Here's how the part is built. I have some questions about the finished solid (model axes, mm). Face numbers are marked on the shaded views. Give positions to 0.01 mm unless a question says otherwise; leave off trailing zeros. Order: outer loops, then holes, each group sorted by start corner. A loop starts at its lowest first (then second) coordinate and runs counter-clockwise, first axis right, second up. Notation, with made-up numbers: (42, 63) -> (85, 63) arc R12 cw to (85, 78) -> close; hole circle Ø8 at (70, 19.25). An arc over 180 degrees is marked (long way). Write each question's results on one line, items separated by ' | '. Start each with the question number.
Q1. Imagine slicing it at A-A, the plane z = 28. Please give me the cut outline in (x, y), then the cut area to 3 significant figures.
Q2. I'm going to push flat-ended pins straight in: pin 1 (1.4 mm diameter, centred on x = 6, y = -11.5, fed in from -Z); pin 2 (3 mm diameter, centred on y = -7, z = -16.5, fed in from -X); pin 3 (6.5 mm diameter, centred on x = 2, z = -47.5, fed in from -Y); pin 4 (1.5 mm diameter, centred on x = -12.5, z = 13, fed in from +Y). Where does each tip first touch, or does it pass through?
Q3. Imagine slicing it at B-B, the plane z = -23.5. Please give me the cut outline in (x, y).
Q4. Thinking about a two-plate mould opening in X: for the marked faces 1 and 2, which applies, pulls with the +X half, pulls with the -X half, needs draft (parallel to the pull), parting line crosses it, or undercut?
Q5. I need wall thicknesses on line 1 along Y through (x, z) = (-19.5, 1); line 2 along X through (y, z) = (-11.75, -6); line 3 along X through (y, z) = (-10, -40.5). Which ranges of each line are inside material? Lowest first, please. Write a range as [from, to].
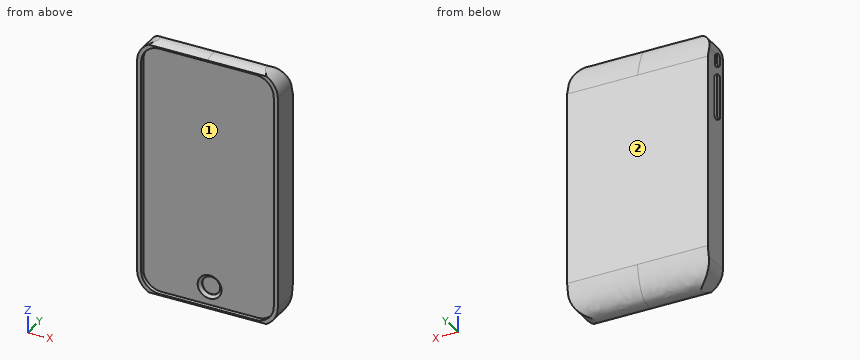
```python
from build123d import *

# Parameters (mm, degrees)
F0_R     = 3.9502971089
F1_DEPTH = 10.668
F2_DEPTH = 12.446
F3_START = 9.144
F3_DEPTH = 9.906
F4_SIZE  = 1.27
F6_DEPTH = 34.798
F8_DEPTH = 31.75


with BuildPart() as f1:
    # F0 (on Front) → F1 (new body)
    with BuildSketch(Plane.XZ):
        with BuildLine():
            Line((-20.9762947197, -56.8147292361), (20.9762947197, -56.8147292361))
            ThreePointArc((20.9762947197, -56.8147292361), (27.8910919329, -53.9505264493), (30.7552947197, -47.0357292361))
            Line((30.7552947197, -47.0357292361), (30.7552947197, 47.0357292361))
            ThreePointArc((30.7552947197, 47.0357292361), (27.8910919329, 53.9505264493), (20.9762947197, 56.8147292361))
            Line((20.9762947197, 56.8147292361), (-20.9762947197, 56.8147292361))
            ThreePointArc((-20.9762947197, 56.8147292361), (-27.8910919329, 53.9505264493), (-30.7552947197, 47.0357292361))
            Line((-30.7552947197, 47.0357292361), (-30.7552947197, -47.0357292361))
            ThreePointArc((-30.7552947197, -47.0357292361), (-27.8910919329, -53.9505264493), (-20.9762947197, -56.8147292361))
        make_face()
        with BuildLine():
            ThreePointArc((20.9762947197, 55.0367310643), (26.6338573688, 52.6932918851), (28.977296548, 47.0357292361))
            Line((28.977296548, 47.0357292361), (28.977296548, -47.0357292361))
            ThreePointArc((28.977296548, -47.0357292361), (26.6338573688, -52.6932918851), (20.9762947197, -55.0367310643))
            Line((20.9762947197, -55.0367310643), (-20.9762947197, -55.0367310643))
            ThreePointArc((-20.9762947197, -55.0367310643), (-26.6338573688, -52.6932918851), (-28.977296548, -47.0357292361))
            Line((-28.977296548, -47.0357292361), (-28.977296548, 47.0357292361))
            ThreePointArc((-28.977296548, 47.0357292361), (-26.6338573688, 52.6932918851), (-20.9762947197, 55.0367310643))
            Line((-20.9762947197, 55.0367310643), (20.9762947197, 55.0367310643))
        make_face(mode=Mode.SUBTRACT)
        with BuildLine():
            Line((28.977296548, -47.0357292361), (28.977296548, 47.0357292361))
            ThreePointArc((28.977296548, 47.0357292361), (26.6338573688, 52.6932918851), (20.9762947197, 55.0367310643))
            Line((20.9762947197, 55.0367310643), (-20.9762947197, 55.0367310643))
            ThreePointArc((-20.9762947197, 55.0367310643), (-26.6338573688, 52.6932918851), (-28.977296548, 47.0357292361))
            Line((-28.977296548, 47.0357292361), (-28.977296548, -47.0357292361))
            ThreePointArc((-28.977296548, -47.0357292361), (-26.6338573688, -52.6932918851), (-20.9762947197, -55.0367310643))
            Line((-20.9762947197, -55.0367310643), (20.9762947197, -55.0367310643))
            ThreePointArc((20.9762947197, -55.0367310643), (26.6338573688, -52.6932918851), (28.977296548, -47.0357292361))
        make_face()
        with Locations((0, -47.0412708819)):
            Circle(F0_R, mode=Mode.SUBTRACT)
        with Locations((0, -47.0412708819)):
            Circle(F0_R)
    extrude(amount=F1_DEPTH)

    # F0 (on Front) → F2 (join)
    with BuildSketch(Plane.XZ):
        with BuildLine():
            Line((-20.9762947197, -56.8147292361), (20.9762947197, -56.8147292361))
            ThreePointArc((20.9762947197, -56.8147292361), (27.8910919329, -53.9505264493), (30.7552947197, -47.0357292361))
            Line((30.7552947197, -47.0357292361), (30.7552947197, 47.0357292361))
            ThreePointArc((30.7552947197, 47.0357292361), (27.8910919329, 53.9505264493), (20.9762947197, 56.8147292361))
            Line((20.9762947197, 56.8147292361), (-20.9762947197, 56.8147292361))
            ThreePointArc((-20.9762947197, 56.8147292361), (-27.8910919329, 53.9505264493), (-30.7552947197, 47.0357292361))
            Line((-30.7552947197, 47.0357292361), (-30.7552947197, -47.0357292361))
            ThreePointArc((-30.7552947197, -47.0357292361), (-27.8910919329, -53.9505264493), (-20.9762947197, -56.8147292361))
        make_face()
        with BuildLine():
            ThreePointArc((20.9762947197, 55.0367310643), (26.6338573688, 52.6932918851), (28.977296548, 47.0357292361))
            Line((28.977296548, 47.0357292361), (28.977296548, -47.0357292361))
            ThreePointArc((28.977296548, -47.0357292361), (26.6338573688, -52.6932918851), (20.9762947197, -55.0367310643))
            Line((20.9762947197, -55.0367310643), (-20.9762947197, -55.0367310643))
            ThreePointArc((-20.9762947197, -55.0367310643), (-26.6338573688, -52.6932918851), (-28.977296548, -47.0357292361))
            Line((-28.977296548, -47.0357292361), (-28.977296548, 47.0357292361))
            ThreePointArc((-28.977296548, 47.0357292361), (-26.6338573688, 52.6932918851), (-20.9762947197, 55.0367310643))
            Line((-20.9762947197, 55.0367310643), (20.9762947197, 55.0367310643))
        make_face(mode=Mode.SUBTRACT)
    extrude(amount=F2_DEPTH)

    # F0 (on Front) → F3 (cut)
    with BuildSketch(Plane.XZ.offset(F3_START)):
        with Locations((0, -47.0412708819)):
            Circle(F0_R)
    extrude(amount=F3_DEPTH, mode=Mode.SUBTRACT)

    # F4
    f4_edges = [f1.edges().sort_by_distance(p)[0] for p in [
        (-3.950297, -10.668, -47.041271),
    ]]
    chamfer(f4_edges, length=F4_SIZE)

    # F5 (on Right) → F6 (cut, symmetric)
    with BuildSketch(Plane.YZ):
        with BuildLine():
            add(Edge.make_bspline(
                [(0, 42.5107741586), (-3.4692891864, 56.6401603672), (-7.0298959202, 56.2049565258), (-9.0349917024, 56.7605619607), (-12.6958908513, 55.4829351604)],
                knots=[0, 0, 0, 0, 0.6298452958, 1, 1, 1, 1], degree=3))
            Line((0, 42.5107741586), (8.7041649967, 42.5107741586))
            Line((8.7041649967, 42.5107741586), (-8.2542682061, 71.9105228782))
            Line((-8.2542682061, 71.9105228782), (-15.3796598309, 57.517234236))
            Line((-15.3796598309, 57.517234236), (-12.6958908513, 55.4829351604))
        make_face()
        with BuildLine():
            Line((6.5665482543, -51.9287921488), (0, -42.5107741586))
            add(Edge.make_bspline(
                [(0, -42.5107741586), (-1.797141266, -55.9935070445), (-8.9519337422, -57.0148502385), (-11.6335880011, -56.1241805553), (-12.6958908513, -55.4829351604)],
                knots=[0, 0, 0, 0, 0.6945936189, 1, 1, 1, 1], degree=3))
            Line((-12.6958908513, -55.4829351604), (-17.793700099, -53.5118058324))
            Line((-17.793700099, -53.5118058324), (-3.83652444, -63.5))
            Line((-3.83652444, -63.5), (6.5665482543, -51.9287921488))
        make_face()
    extrude(amount=F6_DEPTH, both=True, mode=Mode.SUBTRACT)

    # F7 (on Right) → F8 (join)
    with BuildSketch(Plane.YZ):
        with BuildLine():
            Line((-5.6370437269, 18.863574058), (-5.6370437269, 36.3614898325))
            ThreePointArc((-5.6370437269, 36.3614898325), (-6.8880598859, 37.6125059916), (-8.139076045, 36.3614898325))
            Line((-8.139076045, 36.3614898325), (-8.139076045, 18.863574058))
            ThreePointArc((-8.139076045, 18.863574058), (-6.8880598859, 17.6125578989), (-5.6370437269, 18.863574058))
        make_face()
        with BuildLine():
            Line((-5.7985300421, 42.3662230318), (-5.7985300421, 45.7263958405))
            ThreePointArc((-5.7985300421, 45.7263958405), (-6.9122834376, 46.8401492361), (-8.0260368332, 45.7263958405))
            Line((-8.0260368332, 45.7263958405), (-8.0260368332, 42.3662230318))
            ThreePointArc((-8.0260368332, 42.3662230318), (-6.9122834376, 41.2524696362), (-5.7985300421, 42.3662230318))
        make_face()
    extrude(amount=-F8_DEPTH)


solid = f1.part
```
Geometry check:
1) outline: (-31.75, -8.14) -> (-30.76, -8.14) -> (-30.76, -12.45) -> (-28.98, -12.45) -> (-28.98, -10.67) -> (28.98, -10.67) -> (28.98, -12.45) -> (30.76, -12.45) -> (30.76, 0) -> (-30.76, 0) -> (-30.76, -5.64) -> (-31.75, -5.64) -> close | area: 665 mm²
2) pin 1: z = -56.31 | pin 2: x = -30.76 | pin 3: y = -10.67 | pin 4: y = 0
3) outline: (-30.76, -12.45) -> (-28.98, -12.45) -> (-28.98, -10.67) -> (28.98, -10.67) -> (28.98, -12.45) -> (30.76, -12.45) -> (30.76, 0) -> (-30.76, 0) -> close
4) face 1: undercut | face 2: needs draft
5) line 1: [-10.67, 0] | line 2: [-30.76, -28.98], [28.98, 30.76] | line 3: [-30.76, 30.76]
